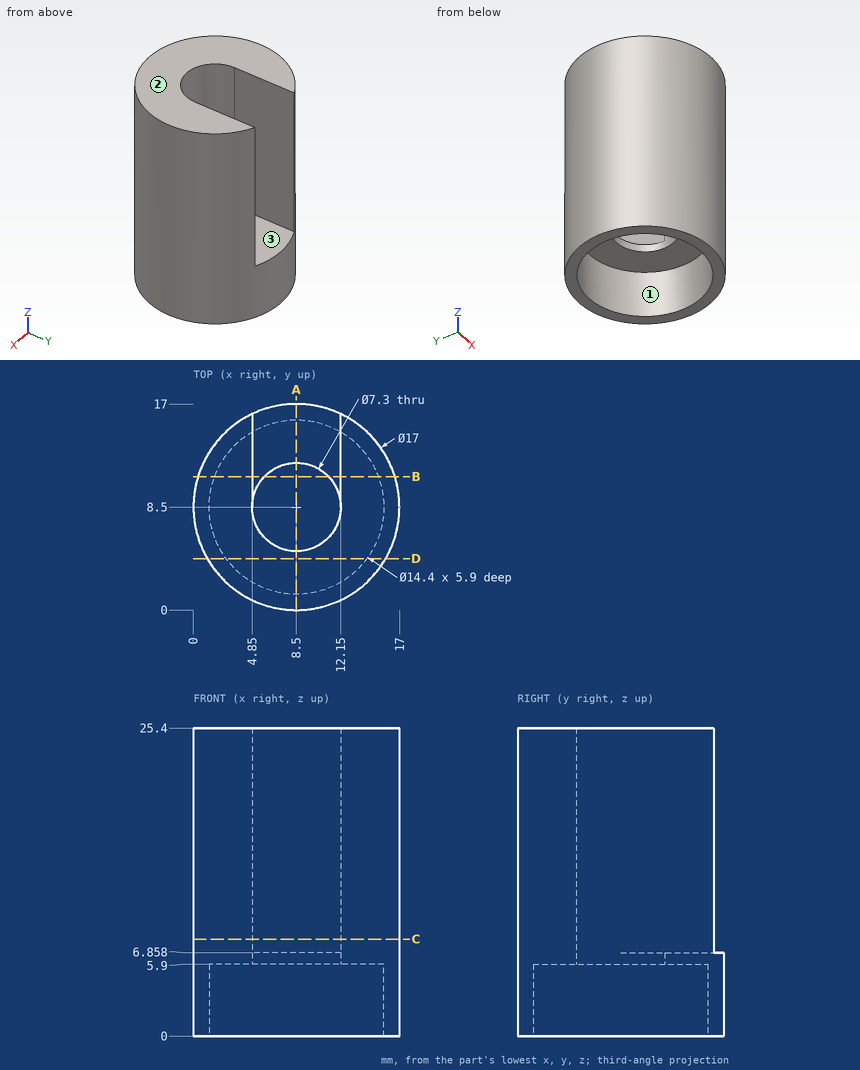
Check sheet for the drawn part. Datum: minimum x, y, z corner. Units: mm. A direction names the side the tool comes from. Coordinates: 2 decimals unless noted, no trailing zeros. Order: outer loops, then holes, each group sorted by start corner. A loop starts at its lowest first (then second) coordinate and runs counter-clockwise, first axis right, second up. Notation, with made-up numbers: M -10,36.5 L 0,36.5 A33 cw 0,72.5 Z; hole C 63,-11.5 d6. An arc over 180 degrees is marked long. One line per question, with ' | ' between items. Start each with the question number.
Item 1: Gauge pin test, flat ends, axial feed: pin 1 (1.5 mm diameter, centred on y = 9.5, z = 16, fed in from -X); pin 2 (3 mm diameter, centred on y = 13.5, z = 19, fed in from +X); pin 3 (4 mm diameter, centred on x = 9.5, y = 5, fed in from -Z). Record the tip position at first contact, or that the pin passes through.
Item 2: Cross-section at B-B on y = 11. Enter the section's corners in (x, z).
Item 3: Cross-section at D-D on y = 4.25. Enter the section's corners in (x, z).
Item 4: Set-up check for the marked faces 1, 2 and 3: record each of +Z, -Z, +X, -X, +Y, -Y from which the full face is reachable in a straight line by a thin tool's end or side.
Item 5: Cross-section at C-C on z = 8. Enter the section's corners in (x, y), then the cut area to 3 significant figures.
Item 6: Cross-section at A-A on x = 8.5. Enter the section's corners in (y, z), then the cut area to 3 significant figures.
Item 7: Material ranges on L1, parallel to X at y = 8.75, z = 3.5; L2, parallel to X at y = 8.5, z = 18.5, recorded low to high. Write a range as [from, to].
Findings:
1) pin 1: stops at x = 0 | pin 2: stops at x = 16.25 | pin 3: stops at z = 5.9
2) outline: M 0.38,0 L 1.75,0 L 1.75,5.9 L 5.84,5.9 L 5.84,6.86 L 4.85,6.86 L 4.85,25.4 L 0.38,25.4 Z; M 11.16,5.9 L 15.25,5.9 L 15.25,0 L 16.62,0 L 16.62,25.4 L 12.15,25.4 L 12.15,6.86 L 11.16,6.86 Z
3) outline: M 1.14,0 L 2.69,0 L 2.69,5.9 L 14.31,5.9 L 14.31,0 L 15.86,0 L 15.86,25.4 L 1.14,25.4 Z
4) face 1: -Z | face 2: +Z, +X, -X, +Y, -Y | face 3: +Z, +Y
5) outline: M 4.85,8.5 L 4.85,16.18 A8.5 ccw long 12.15,16.18 L 12.15,8.5 A3.65 cw Z | area: 146 mm²
6) outline: M 0,0 L 1.3,0 L 1.3,5.9 L 4.85,5.9 L 4.85,25.4 L 0,25.4 Z; M 12.15,5.9 L 15.7,5.9 L 15.7,0 L 17,0 L 17,6.86 L 12.15,6.86 Z | area: 115 mm²
7) L1: x = [0, 1.3], [15.7, 17] | L2: x = [0, 4.85], [12.15, 17]
